Check sheet for the modelled part. Datum: model origin and axes. Units: mm. Face numbers are marked on the shaded views. A direction names the side the tool comes from. Round coordinates to 2 decimals unless told otherwise and drop trailing zeros. Order: outer loops, then holes, each group sorted by start corner. A loop starts at its lowest first (then second) coordinate and runs counter-clockwise, first axis right, second up. Notation, with made-up numbers: (5.5, -19.75) -> (55.5, -19.75) arc R22 ccw to (55.5, 12.25) -> close; hole circle Ø1 at (46.5, 44). An arc over 180 degrees is marked (long way). Answer in a Markdown table with one row per item.
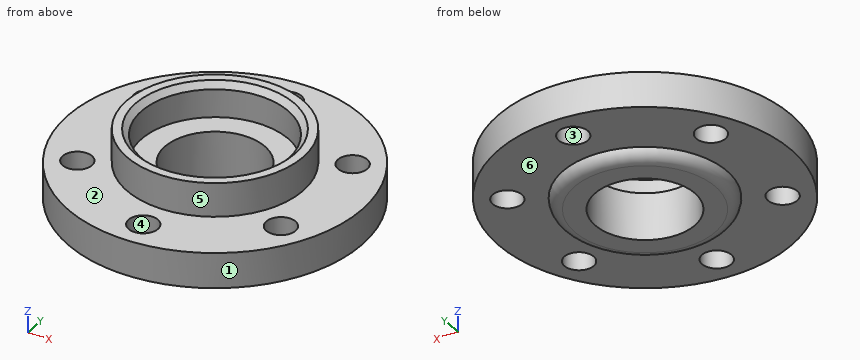
from build123d import *

# Parameters (mm, degrees)
SKETCH1_R                = 25
BOSS_EXTRUDE1_DEPTH      = 6
SKETCH2_R                = 15
SKETCH2_R_2              = 12.5
BOSS_EXTRUDE2_DEPTH      = 5.75
SKETCH3_R                = 14
BOSS_EXTRUDE3_DEPTH      = 2
FILLET1_R                = 2
CHAMFER1_SIZE            = 1
F_5_0_5_DIAMETER_HOLE1_D = 5
CIRPATTERN1_COUNT        = 6
SKETCH10_R               = 8.5
CUT_EXTRUDE1_DEPTH       = 38.934977264


with BuildPart() as part:
    # Sketch1 → Boss-Extrude1 (new body)
    with BuildSketch(Plane.XY):
        Circle(SKETCH1_R)
    extrude(amount=BOSS_EXTRUDE1_DEPTH)

    # Sketch2 → Boss-Extrude2 (add)
    with BuildSketch(Plane.XY.offset(6)):
        Circle(SKETCH2_R)
        Circle(SKETCH2_R_2, mode=Mode.SUBTRACT)
    extrude(amount=BOSS_EXTRUDE2_DEPTH)

    # Sketch3 → Boss-Extrude3 (add)
    with BuildSketch(Plane(origin=(0, 0, 0), x_dir=(-1, 0, 0), z_dir=(0, 0, -1))):
        with Locations(Location((0, 0, 0), (0, 0, 180))):
            Circle(SKETCH3_R)
    extrude(amount=BOSS_EXTRUDE3_DEPTH)

    # Fillet1
    fillet1_edges = [part.edges().sort_by_distance(p)[0] for p in [
        (-14, 0, -2),
    ]]
    fillet(fillet1_edges, radius=FILLET1_R - 0.0001)  # a hair under: the kernel refuses the full size

    # Chamfer1
    chamfer1_edges = [part.edges().sort_by_distance(p)[0] for p in [
        (-12.5, 0, 11.75),
    ]]
    chamfer(chamfer1_edges, length=CHAMFER1_SIZE)

    # Ø5.0 (5) Diameter Hole1 (through all)
    with Locations(Plane(origin=(0, 0, 0), x_dir=(-1, 0, 0), z_dir=(0, 0, -1))):
        with Locations((0, 20)):
            f_5_0_5_diameter_hole1 = Hole(F_5_0_5_DIAMETER_HOLE1_D / 2)

    # CirPattern1: Ø5.0 (5) Diameter Hole1 ×6 about axis
    cirpattern1_axis = Axis((0, 0, 0), (0, 0, 1))
    for i in range(1, CIRPATTERN1_COUNT):
        add(f_5_0_5_diameter_hole1.rotate(cirpattern1_axis, i * 360 / CIRPATTERN1_COUNT), mode=Mode.SUBTRACT)

    # Sketch10 → Cut-Extrude1 (cut, through all)
    with BuildSketch(Plane(origin=(0, 0, -2), x_dir=(-1, 0, 0), z_dir=(0, 0, -1))):
        Circle(SKETCH10_R)
    extrude(amount=-CUT_EXTRUDE1_DEPTH, mode=Mode.SUBTRACT)


solid = part.part
Item 1: Cross-section at B-B (x = 0). State how many separate pieces and enclosed holes the cut face has, and give its area (3 significant figures).
Result sheet:
| item | result |
|---|---|
| separate pieces | 4 |
| enclosed holes | 0 |
| area | 186 mm^2 |
Item 2: Scan lines: line 1 (Y direction, x = 0, z = 1.75); line 2 (Y direction, x = 17, z = 1.25); line 3 (Y direction, x = 16.5, z = 0.75). Record each from-to range of solid material in increasing order. Write a range as [from, to].
Result sheet:
| item | result |
|---|---|
| line 1 | y = [-25, -22.5], [-17.5, -8.5], [8.5, 17.5], [22.5, 25] |
| line 2 | y = [-18.33, -12.48], [-7.52, 7.52], [12.48, 18.33] |
| line 3 | y = [-18.78, -12.36], [-7.64, 7.64], [12.36, 18.78] |
Item 3: Depth check by flat-ended pin: P1, Ø20, axis at x = 0, y = 0, coming from the +Z side; P2, Ø5, axis at y = -0.5, z = 9.5, coming from the -X side; P3, Ø6.5, axis at x = 0, y = 20, coming from the -Z side. Enter the tip coordinate at first touch or a pass-through.
Result sheet:
| item | result |
|---|---|
| P1 | stops at z = 6 |
| P2 | stops at x = -15 |
| P3 | stops at z = 0 |
Item 4: Set-up check for the marked faces 4, 5 and 6: record each of +Z, -Z, +X, -X, +Y, -Y from which the full face is reachable in a straight line by a thin tool's end or side.
Result sheet:
| item | result |
|---|---|
| face 4 | +Z, -Z |
| face 5 | +Z |
| face 6 | -Z |
Item 5: Cross-section at D-D (z = 7.75). Record the boundary of the cut face in (x, y).
Result sheet:
| item | result |
|---|---|
| outline | circle Ø30 at (0, 0); hole circle Ø25 at (0, 0) |
Item 6: Cross-section at C-C (z = 2). Record the boundary of the cut face in (x, y), and give its area (3 significant figures).
Result sheet:
| item | result |
|---|---|
| outline | circle Ø50 at (0, 0); hole circle Ø5 at (-17.32, -10); hole circle Ø5 at (-17.32, 10); hole circle Ø17 at (0, 0); hole circle Ø5 at (0, -20); hole circle Ø5 at (0, 20); hole circle Ø5 at (17.32, -10); hole circle Ø5 at (17.32, 10) |
| area | 1,620 mm^2 |
Item 7: Mould release check, pull along X, two halves, no side actions. Record for the marked faces 1, 2 and 3: pulls with the +X half, pulls with the -X half, needs draft (parallel to the pull), parting line crosses it, or undercut.
Result sheet:
| item | result |
|---|---|
| face 1 | parting line crosses it |
| face 2 | needs draft |
| face 3 | undercut |
Item 8: Cross-section at A-A (y = -20). Record the boundary of the cut face in (x, z).
Result sheet:
| item | result |
|---|---|
| outline | (-15, 0) -> (-2.5, 0) -> (-2.5, 6) -> (-15, 6) -> close; (2.5, 0) -> (15, 0) -> (15, 6) -> (2.5, 6) -> close |
